```python
from build123d import *

# Parameters (mm, degrees)
SKETCH1_W          = 85.5
SKETCH1_H          = 19
SKETCH2_R          = 5
CUT_EXTRUDE1_DEPTH = 446.882271457


with BuildPart() as part:
    # Sketch1 → Revolve1 (revolve)
    with BuildSketch(Plane(origin=(0, 0, 0), x_dir=(0, 0, -1), z_dir=(1, 0, 0)), mode=Mode.PRIVATE) as revolve1_sk:
        with Locations((-272.25, -18.279378005)):
            Rectangle(SKETCH1_W, SKETCH1_H)
    revolve(revolve1_sk.sketch.rotate(Axis((0, -6970.88671751, 0), (0, 1, 0)), 180), axis=Axis((0, -6970.88671751, 0), (0, 1, 0)))

    # Sketch2 → Cut-Extrude1 (cut, through all)
    with BuildSketch(Plane(origin=(0, -8.779378005, 0), x_dir=(1, 0, 0), z_dir=(0, 1, 0))):
        with Locations(Location((0, 240, 0), (0, 0, 270))):
            Circle(SKETCH2_R)
        with Locations(Location((169.705627485, 169.705627485, 0), (0, 0, 270))):
            Circle(SKETCH2_R)
        with Locations(Location((240, 0, 0), (0, 0, 270))):
            Circle(SKETCH2_R)
        with Locations(Location((169.705627485, -169.705627485, 0), (0, 0, 270))):
            Circle(SKETCH2_R)
        with Locations(Location((0, -240, 0), (0, 0, 270))):
            Circle(SKETCH2_R)
        with Locations(Location((-169.705627485, -169.705627485, 0), (0, 0, 270))):
            Circle(SKETCH2_R)
        with Locations(Location((-240, 0, 0), (0, 0, 270))):
            Circle(SKETCH2_R)
        with Locations(Location((-169.705627485, 169.705627485, 0), (0, 0, 270))):
            Circle(SKETCH2_R)
    extrude(amount=-CUT_EXTRUDE1_DEPTH, mode=Mode.SUBTRACT)


solid = part.part
```
Source: CAD feature listing. Evaluate the final solid. Frame: model axes, mm. Coordinates: 2 decimals unless noted, no trailing zeros. Write each loop counter-clockwise with the first axis right and the second up, starting at its lowest first coordinate (ties: lowest second). Pieces come first, ordered by that corner, then holes. Notation, with made-up numbers: M 84.25,-10.75 L 96.25,-10.75 A33 ccw 96.25,25.25 Z; hole C -10.5,75 d9. An arc over 180 degrees is marked long. Answer as a JSON object with one key per item and string values.
1. Draft query along X for faces 1 (the cylindrical face through (307.51, -18.15, 68.29)), 2 (the flat face through (232, -8.779, -22)), 3 (the cylindrical face through (224.043, -18.146, 49.751)). Return one class per face: released by +X, released by -X, zero draft, split by the parting line, or undercut.
Evaluation:
{"face 1": "split by the parting line", "face 2": "zero draft", "face 3": "undercut"}
2. Ray query, L1, parallel to X at y = -21.5, z = 0; L2, parallel to X at y = -18.5, z = -2.5; L3, parallel to X at y = -11, z = -77. Return the intervals inside material, ascending.
Evaluation:
{"L1": "-315 to -245, -235 to -229.5, 229.5 to 235, 245 to 315", "L2": "-314.99 to -244.33, -235.67 to -229.49, 229.49 to 235.67, 244.33 to 314.99", "L3": "-305.44 to -216.2, 216.2 to 305.44"}
3. Cut plane B-B on x = 143. Output: boundary loops of the cut face in (y, z).
Evaluation:
{"outline": "M -27.78,-280.67 L -8.78,-280.67 L -8.78,-179.5 L -27.78,-179.5 Z; M -27.78,179.5 L -8.78,179.5 L -8.78,280.67 L -27.78,280.67 Z"}
4. Cut plane D-D on x = 270. Output: boundary loops of the cut face in (y, z).
Evaluation:
{"outline": "M -27.78,-162.25 L -8.78,-162.25 L -8.78,162.25 L -27.78,162.25 Z"}
5. Cut plane A-A on z = 71.5. Output: boundary loops of the cut face in (x, y).
Evaluation:
{"outline": "M -306.78,-27.78 L -218.08,-27.78 L -218.08,-8.78 L -306.78,-8.78 Z; M 218.08,-27.78 L 306.78,-27.78 L 306.78,-8.78 L 218.08,-8.78 Z"}
6. Contact query for flat-ended pins moving along their axis: P1, Ø16, axis at x = -169.71, z = 169.71, coming from the -Y side; P2, Ø10, axis at x = -108, y = -18, coming from the +Z side; P3, Ø5, axis at x = -117.5, y = -13, coming from the +Z side; P4, Ø6, axis at x = -76, y = -13.5, coming from the -Z side. Output: stop coordinate, or through.
Evaluation:
{"P1": "y = -27.78", "P2": "z = 297.68", "P3": "z = 293.26", "P4": "z = -306.42"}
7. Cut plane C-C on y = -23. State how many separate pieces and enclosed holes the cut face has, plus the area to 3 significant figures.
Evaluation:
{"separate pieces": "1", "enclosed holes": "9", "area": "146,000 mm^2"}
